```python
from build123d import *

# Parameters (mm, degrees)
IZIM1_R                     = 4.45
Y_KSEKLIK_EKSTR_ZYON1_DEPTH = 5.6
IZIM2_R                     = 0.85
IZIM2_R_2                   = 4.45
Y_KSEKLIK_EKSTR_ZYON3_DEPTH = 2.3
RADYUS1_R                   = 0.5
IZIM3_R                     = 2.95
KES_EKSTR_ZYON1_DEPTH       = 1.05
IZIM7_R                     = 4.65
IZIM7_R_2                   = 3.335
KES_EKSTR_ZYON3_DEPTH       = 1.05
IZIM8_R                     = 2.95
KES_EKSTR_ZYON5_DEPTH       = 1.05
IZIM9_R                     = 2.95
Y_KSEKLIK_EKSTR_ZYON4_DEPTH = 1.05
IZIM10_R                    = 1.5
KES_EKSTR_ZYON6_DEPTH       = 8.05
IZIM11_R                    = 2.68
KES_EKSTR_ZYON7_DEPTH       = 3.5
KES_EKSTR_ZYON10_DEPTH      = 12.5
DAIRESEL_KAPLAMA1_COUNT     = 24


with BuildPart() as part:
    # Çizim1 → Yükseklik-Ekstrüzyon1 (new body)
    with BuildSketch(Plane.XY):
        Circle(IZIM1_R)
    extrude(amount=Y_KSEKLIK_EKSTR_ZYON1_DEPTH)

    # Çizim2 → Yükseklik-Ekstrüzyon3 (add)
    with BuildSketch(Plane.XY.offset(5.6)):
        with BuildLine():
            Line((-4.370037185, 4.22), (-4.370301647, 4.22))
            Line((-4.370301647, 4.22), (-16.5, 2.6))
            ThreePointArc((-16.5, 2.6), (-19.1, 0), (-16.5, -2.6))
            Line((-16.5, -2.6), (-4.369998027, -4.22004055))
            ThreePointArc((-4.369998027, -4.22004055), (0, -6.075), (4.369998027, -4.22004055))
            Line((4.369998027, -4.22004055), (16.5, -2.6))
            ThreePointArc((16.5, -2.6), (19.1, 0), (16.5, 2.6))
            Line((16.5, 2.6), (4.370301647, 4.22))
            Line((4.370301647, 4.22), (4.370037185, 4.22))
            ThreePointArc((4.370037185, 4.22), (0, 6.075), (-4.370037185, 4.22))
        make_face()
        with Locations((-16.5, 0)):
            Circle(IZIM2_R, mode=Mode.SUBTRACT)
        with Locations((-13.5, 0)):
            Circle(IZIM2_R, mode=Mode.SUBTRACT)
        with Locations((-10.5, 0)):
            Circle(IZIM2_R, mode=Mode.SUBTRACT)
        with Locations((-7.5, 0)):
            Circle(IZIM2_R, mode=Mode.SUBTRACT)
        Circle(IZIM2_R_2, mode=Mode.SUBTRACT)
        with Locations((7.5, 0)):
            Circle(IZIM2_R, mode=Mode.SUBTRACT)
        with Locations((10.5, 0)):
            Circle(IZIM2_R, mode=Mode.SUBTRACT)
        with Locations((13.5, 0)):
            Circle(IZIM2_R, mode=Mode.SUBTRACT)
        with Locations((16.5, 0)):
            Circle(IZIM2_R, mode=Mode.SUBTRACT)
    extrude(amount=-Y_KSEKLIK_EKSTR_ZYON3_DEPTH)

    # Radyus1
    radyus1_edges = [part.edges().sort_by_distance(p)[0] for p in [
        (-4.369998027, -4.22004055, 4.45),
        (4.369998027, -4.22004055, 4.45),
    ]]
    fillet(radyus1_edges, radius=RADYUS1_R)

    # Çizim3 → Kes-Ekstrüzyon1 (cut)
    with BuildSketch(Plane(origin=(0, 0, 0), x_dir=(-1, 0, 0), z_dir=(0, 0, -1))):
        Circle(IZIM3_R)
    extrude(amount=-KES_EKSTR_ZYON1_DEPTH, mode=Mode.SUBTRACT)

    # Çizim7 → Kes-Ekstrüzyon3 (cut)
    with BuildSketch(Plane.XY.offset(5.6)):
        Circle(IZIM7_R)
        Circle(IZIM7_R_2, mode=Mode.SUBTRACT)
    extrude(amount=-KES_EKSTR_ZYON3_DEPTH, mode=Mode.SUBTRACT)

    # Çizim8 → Kes-Ekstrüzyon5 (cut)
    with BuildSketch(Plane.XY.offset(5.6)):
        with Locations(Location((0, 0, 0), (0, 0, 180))):
            Circle(IZIM8_R)
    extrude(amount=-KES_EKSTR_ZYON5_DEPTH, mode=Mode.SUBTRACT)

    # Çizim9 → Yükseklik-Ekstrüzyon4 (add)
    with BuildSketch(Plane(origin=(0, 0, 1.05), x_dir=(-1, 0, 0), z_dir=(0, 0, -1))):
        with Locations(Location((0, 0, 0), (0, 0, 180))):
            Circle(IZIM9_R)
    extrude(amount=Y_KSEKLIK_EKSTR_ZYON4_DEPTH)

    # Çizim10 → Kes-Ekstrüzyon6 (cut)
    with BuildSketch(Plane.XY.offset(4.55)):
        Circle(IZIM10_R)
    extrude(amount=-KES_EKSTR_ZYON6_DEPTH, mode=Mode.SUBTRACT)

    # Çizim11 → Kes-Ekstrüzyon7 (cut)
    with BuildSketch(Plane(origin=(0, 0, 0), x_dir=(-1, 0, 0), z_dir=(0, 0, -1))):
        Circle(IZIM11_R)
    extrude(amount=-KES_EKSTR_ZYON7_DEPTH, mode=Mode.SUBTRACT)

    # Çizim12 → Kes-Ekstrüzyon10 (cut)
    with BuildSketch(Plane(origin=(0, 0, 3.5), x_dir=(-1, 0, 0), z_dir=(0, 0, -1))):
        with BuildLine():
            Line((-2.000304803, 2.302451019), (-1.938517615, 1.850553824))
            ThreePointArc((-1.938517615, 1.850553824), (-1.686954029, 2.082447143), (-1.407896467, 2.280400741))
            Line((-1.407896467, 2.280400741), (-1.837127974, 2.434637716))
            ThreePointArc((-1.837127974, 2.434637716), (-1.919854398, 2.369949174), (-2.000304803, 2.302451019))
        make_face()
    kes_ekstr_zyon10 = extrude(amount=KES_EKSTR_ZYON10_DEPTH, mode=Mode.SUBTRACT)

    # Dairesel Kaplama1: Kes-Ekstrüzyon10 ×24 about axis
    dairesel_kaplama1_axis = Axis((0, 0, 0), (0, 0, 1))
    for i in range(1, DAIRESEL_KAPLAMA1_COUNT):
        add(kes_ekstr_zyon10.rotate(dairesel_kaplama1_axis, i * 360 / DAIRESEL_KAPLAMA1_COUNT), mode=Mode.SUBTRACT)


solid = part.part
```
Design review of the part built by this model. Coordinates are the model's own, in mm. A direction names the side the tool comes from. Round coordinates to 2 decimals unless told otherwise and drop trailing zeros. Write each loop counter-clockwise with the first axis right and the second up, starting at its lowest first coordinate (ties: lowest second). Pieces come first, ordered by that corner, then holes. Notation, with made-up numbers: (45.25, 53) -> (56.25, 53) arc R32 ccw to (56.25, 79) -> close; hole circle Ø6 at (46, 20.25). An arc over 180 degrees is marked (long way). Write item = value, one per line. Start each with the question number.
1) Wall thickness on probe 1 along Y at (x, z) = (0, 5.15) (3 decimals); probe 2 along Y at (x, z) = (0, 4) (3 decimals); probe 3 along Y at (x, z) = (13.5, 3.55): over which ranges is each line inside the solid? List them lowest first. Write a range as from..to.
2) Tool access review of faces 1 (the face through (0.068, 6.075, 4.466)), 2 (the face through (2.947, -0.13, 5.082)): name each direction out of +Z, -Z, +X, -X, +Y, -Y from which nothing blocks a thin tool from reaching the whole face with its end or side.
3) Take a section at B-B, the plane x = -7.5. State the section outline as (y, z) points.
4) Take a section at C-C, the plane x = -13.5. State the section outline as (y, z) points, plus the area to 3 significant figures.
5) Clearance check with flat-ended pins moving along their axes: pin 1 (1.5 mm diameter, centred on x = -13.5, y = 0, fed in from -Z); pin 2 (2 mm diameter, centred on x = -7.5, y = 0, fed in from -Z); pin 3 (3.5 mm diameter, centred on x = 0, y = 0, fed in from +Z). State where each tip first meets the part, or that it passes through.
6) Take a section at A-A, the plane z = 5.2. Count the separate pieces of the cut face and the enclosed holes in it, plus the area to 3 significant figures.
7) Mouldability with a two-part tool opening along Y and no side actions: class faces 3 (the face through (-12.715, -0.326, 4.466)), 4 (the face through (-19.1, 0.1, 4.5)), 5 (the face through (-10.35, 3.42, 4.47)) as +Y half, -Y half, draft (parallel to the pull), parting line (faces both ways), or undercut.
Results list:
q1.probe_1 = -6.075..-4.65, -3.335..-2.95, 2.95..3.335, 4.65..6.075
q1.probe_2 = -6.075..-1.5, 1.5..6.075
q1.probe_3 = -3..-0.85, 0.85..3
q2.face_1 = +Z, -Z, +Y
q2.face_2 = +Z
q3.outline = (-3.8, 3.3) -> (-0.85, 3.3) -> (-0.85, 5.6) -> (-3.8, 5.6) -> close; (0.85, 3.3) -> (3.8, 3.3) -> (3.8, 5.6) -> (0.85, 5.6) -> close
q4.outline = (-3, 3.3) -> (-0.85, 3.3) -> (-0.85, 5.6) -> (-3, 5.6) -> close; (0.85, 3.3) -> (3, 3.3) -> (3, 5.6) -> (0.85, 5.6) -> close
q4.area = 9.89 mm²
q5.pin_1 = through
q5.pin_2 = 3.3
q5.pin_3 = 4.55
q6.separate_pieces = 2
q6.enclosed_holes = 10
q6.area = 204 mm²
q7.face_3 = undercut
q7.face_4 = parting line
q7.face_5 = +Y half
